Input: part model. Units: mm. Frame: model coordinates. A direction names the side the tool comes from. Coordinates: 2 decimals unless noted, no trailing zeros. Loops run counter-clockwise (first coordinate to the right, second up) from the corner with the lowest first, then second, coordinate; pieces in that order, holes last. Notation, with made-up numbers: (67.25, 69) -> (101.25, 69) arc R4 ccw to (101.25, 75) -> close; hole circle Ø4 at (14, 74.5). An arc over 180 degrees is marked (long way). Put each result on its own line as item: value. Start each with the question number.
1) Material intervals for L1, parallel to Y at x = 82.5, z = 35; L2, parallel to X at y = -15.5, z = 30; L3, parallel to X at y = 43, z = 32, sorted ascending.
2) Cut plane D-D (x = 156.5). Return the cut outline in (y, z), plus the area to 3 significant figures.
3) Cut plane B-B (z = 26.5). Return the cut outline in (x, y), plus the area to 3 significant figures.
4) Pull-direction query (Y, two-part tool) for faces 1 (the flat face through (12, 2, 22.092)), 2 (the cylindrical face through (62.707, 7.706, 39.885)), 3 (the cylindrical face through (123.83, 0.82, 32.07)), 4 (the flat face through (37, -42.729, 39)); classes: pulls with the +Y half, pulls with the -Y half, needs draft (parallel to the pull), parting line crosses it, or undercut.
5) Cut plane A-A (y = 0). Return the cut outline in (x, z).
6) Contact query for flat-ended pins moving along their axis: P1, Ø10, axis at x = 85, z = 41.5, coming from the +Y side; P2, Ø10, axis at y = -0.5, z = 52, coming from the +X side; P3, Ø15.5, axis at x = 164, z = 30, coming from the -Y side. Output: stop coordinate, or through.
7) Cut plane C-C (z = 46.5). Return the cut outline in (x, y).
8) Set-up query: faces 5 (the flat face through (143, -31.032, 32)), 6 (the flat face through (143, 20.787, 32)), 7 (the flat face through (37, 48.711, 39)), 8 (the flat face through (127, -11, 41.772)). Return all of +Z, -Z, +X, -X, +Y, -Y with unobstructed straight access to the full face (end or side cutting, diameter ignored); none if empty.
from build123d import *

# Parameters (mm, degrees)
F0_W     = 91.44
F0_H     = 35.094067
F1_DEPTH = 74.66243
F2_R     = 25.655488
F3_DEPTH = 59.964648
F4_W     = 51.819967
F4_H     = 19.67985
F5_DEPTH = 138.002442
F6_R     = 18.602683
F7_DEPTH = 87.077601


with BuildPart() as f1:
    # F0 (on Right) → F1 (new body)
    with BuildSketch(Plane.YZ):
        with Locations((2.991382, 39.639005)):
            Rectangle(F0_W, F0_H)
    extrude(amount=F1_DEPTH)

    # F2 (on face) → F3 (cut)
    with BuildSketch(Plane.XY.offset(57.186039)):
        with Locations((38.235784, 0)):
            Circle(F2_R)
    extrude(amount=-F3_DEPTH, mode=Mode.SUBTRACT)

    # F4 (on face) → F5 (join)
    with BuildSketch(Plane.YZ.offset(74.66243)):
        with Locations((-5.12249, 31.931897)):
            Rectangle(F4_W, F4_H)
    extrude(amount=F5_DEPTH)

    # F6 (on face) → F7 (cut)
    with BuildSketch(Plane.XY.offset(41.771822)):
        with Locations((142.413676, 0)):
            Circle(F6_R)
    extrude(amount=-F7_DEPTH, mode=Mode.SUBTRACT)


solid = f1.part
Results found:
1. L1: y = -31.03 to 20.79
1. L2: x = 0 to 17.79, 58.68 to 132.13, 152.7 to 212.66
1. L3: x = 0 to 74.66
2. outline: (-31.03, 22.09) -> (-12.15, 22.09) -> (-12.15, 41.77) -> (-31.03, 41.77) -> close; (12.15, 22.09) -> (20.79, 22.09) -> (20.79, 41.77) -> (12.15, 41.77) -> close
2. area: 542 mm2
3. outline: (0, -42.73) -> (74.66, -42.73) -> (74.66, -31.03) -> (212.66, -31.03) -> (212.66, 20.79) -> (74.66, 20.79) -> (74.66, 48.71) -> (0, 48.71) -> close; hole circle Ø51.31 at (38.24, 0); hole circle Ø37.21 at (142.41, 0)
3. area: 10,800 mm2
4. face 1: needs draft
4. face 2: undercut
4. face 3: undercut
4. face 4: pulls with the -Y half
5. outline: (0, 22.09) -> (12.58, 22.09) -> (12.58, 57.19) -> (0, 57.19) -> close; (63.89, 22.09) -> (123.81, 22.09) -> (123.81, 41.77) -> (74.66, 41.77) -> (74.66, 57.19) -> (63.89, 57.19) -> close; (161.02, 22.09) -> (212.66, 22.09) -> (212.66, 41.77) -> (161.02, 41.77) -> close
6. P1: stops at y = 20.79
6. P2: stops at x = 74.66
6. P3: stops at y = -31.03
7. outline: (0, -42.73) -> (74.66, -42.73) -> (74.66, 48.71) -> (0, 48.71) -> close; hole circle Ø51.31 at (38.24, 0)
8. face 5: +Z, -Z, +X, -Y
8. face 6: +Z, -Z, +X, +Y
8. face 7: +Z, -Z, +X, -X, +Y
8. face 8: +Z, +X, +Y, -Y
